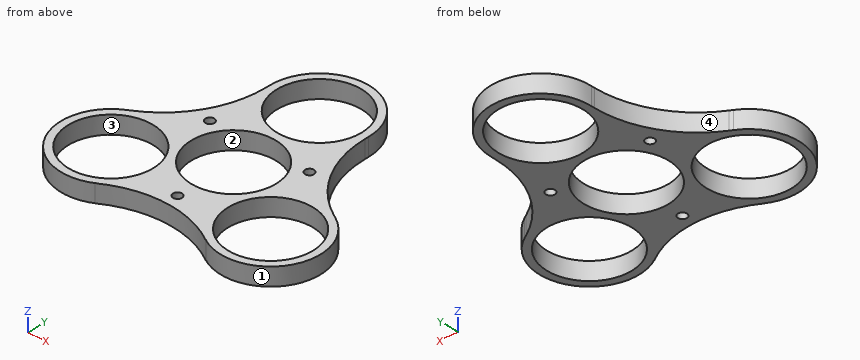
```python
from build123d import *

# Parameters (mm, degrees)
SKETCH1_R           = 11.9
SKETCH1_R_2         = 1.25
BOSS_EXTRUDE1_DEPTH = 2.5


with BuildPart() as part:
    # Sketch1 → Boss-Extrude1 (new, symmetric)
    with BuildSketch(Plane.XY):
        with BuildLine():
            Line((13.998405034, 25.788679153), (13.997620563, 24.84501718))
            ThreePointArc((13.997620563, 24.84501718), (17.915653408, 10.264281088), (28.632025365, -0.370953675))
            Line((28.632025365, -0.370953675), (29.451770584, -0.838410955))
            ThreePointArc((29.451770584, -0.838410955), (34.50421589, -20.231771272), (14.992592767, -24.806286663))
            Line((14.992592767, -24.806286663), (15.585568871, -25.184186379))
            ThreePointArc((15.585568871, -25.184186379), (0, -20.640065896), (-15.585568871, -25.184186379))
            Line((-15.585568871, -25.184186379), (-14.992592767, -24.806286663))
            ThreePointArc((-14.992592767, -24.806286663), (-34.504073282, -20.232007658), (-29.452250217, -0.838684477))
            Line((-29.452250217, -0.838684477), (-28.632523434, -0.371194867))
            ThreePointArc((-28.632523434, -0.371194867), (-17.951478652, 10.204474397), (-13.999324478, 24.706542367))
            Line((-13.999324478, 24.706542367), (-13.995629252, 25.650197431))
            ThreePointArc((-13.995629252, 25.650197431), (-0.069254769, 39.999828705), (13.998405034, 25.788679153))
        make_face()
        Circle(SKETCH1_R, mode=Mode.SUBTRACT)
        with Locations((0, 26)):
            Circle(SKETCH1_R, mode=Mode.SUBTRACT)
        with Locations((22.516660498, -13)):
            Circle(SKETCH1_R, mode=Mode.SUBTRACT)
        with Locations((-22.516660498, -13)):
            Circle(SKETCH1_R, mode=Mode.SUBTRACT)
        with Locations((13.983602476, 7.982266036)):
            Circle(SKETCH1_R_2, mode=Mode.SUBTRACT)
        with Locations((0, -17)):
            Circle(SKETCH1_R_2, mode=Mode.SUBTRACT)
        with Locations((-14.064993078, 7.936657484)):
            Circle(SKETCH1_R_2, mode=Mode.SUBTRACT)
    extrude(amount=BOSS_EXTRUDE1_DEPTH, both=True)


solid = part.part
```
Could you check a few things on this model? Use its own coordinates, in mm. Face numbers are marked on the shaded views. Round coordinates to 2 decimals unless told otherwise and drop trailing zeros. Loops run counter-clockwise (first coordinate to the right, second up) from the corner with the lowest first, then second, coordinate; pieces in that order, holes last. Notation, with made-up numbers: (70, -31.5) - (75, -31.5) arc R24 cw to (75, -12.5) - close; hole circle Ø5 at (12.25, -36). An arc over 180 degrees is marked (long way). Answer in a Markdown table with one row per item. Add a question column.
(1) If we section it at A-A (x = 0): Please give me the cut outline in (y, z), plus the area to 3 significant figures.
(2) I need wall thicknesses on line 1 along Y through (x, z) = (6, -0.85); line 2 along Y through (x, z) = (0, 1.2); line 3 along Y through (x, z) = (-9, -2.2). Which ranges of each line are inside material? Lowest first, please.
(3) If we mould it in two halves opening along Y, with no side actions, what happens to the marked faces 1, 2, 3 and 4? For each: pulls with the +Y half, pulls with the -Y half, needs draft (parallel to the pull), parting line crosses it, or undercut.
(4) If we section it at D-D (x = 22): Please give me the cut outline in (y, z), plus the area to 3 significant figures.
(5) If we section it at B-B (y = -13): Please give me the cut outline in (x, z), plus the area to 3 significant figures.
(6) If we section it at C-C (y = -3): Please give me the cut outline in (x, z).
(7) I'm going to push flat-ended pins straight in: pin 1 (21.5 mm diameter, centred on x = 22.52, y = -13, fed in from +Z); pin 2 (3 mm diameter, centred on y = 23, z = -2, fed in from -X). Where does each tip first touch, or does it pass through?
Model answer:
| question | item | result |
|---|---|---|
| 1 | outline | (-20.64, -2.5) - (-18.25, -2.5) - (-18.25, 2.5) - (-20.64, 2.5) - close; (-15.75, -2.5) - (-11.9, -2.5) - (-11.9, 2.5) - (-15.75, 2.5) - close; (11.9, -2.5) - (14.1, -2.5) - (14.1, 2.5) - (11.9, 2.5) - close; (37.9, -2.5) - (40, -2.5) - (40, 2.5) - (37.9, 2.5) - close |
| 1 | area | 52.7 mm² |
| 2 | line 1 | y = -21.27 to -10.28, 10.28 to 15.72, 36.28 to 38.65 |
| 2 | line 2 | y = -20.64 to -18.25, -15.75 to -11.9, 11.9 to 14.1, 37.9 to 40 |
| 2 | line 3 | y = -22.07 to -7.79, 7.79 to 18.21, 33.79 to 36.72 |
| 3 | face 1 | parting line crosses it |
| 3 | face 2 | undercut |
| 3 | face 3 | undercut |
| 3 | face 4 | pulls with the +Y half |
| 4 | outline | (-26.99, -2.5) - (-24.89, -2.5) - (-24.89, 2.5) - (-26.99, 2.5) - close; (-1.11, -2.5) - (4.82, -2.5) - (4.82, 2.5) - (-1.11, 2.5) - close |
| 4 | area | 40.2 mm² |
| 5 | outline | (-36.52, -2.5) - (-34.42, -2.5) - (-34.42, 2.5) - (-36.52, 2.5) - close; (-10.62, -2.5) - (10.62, -2.5) - (10.62, 2.5) - (-10.62, 2.5) - close; (34.42, -2.5) - (36.52, -2.5) - (36.52, 2.5) - (34.42, 2.5) - close |
| 5 | area | 127 mm² |
| 6 | outline | (-32.31, -2.5) - (-28.97, -2.5) - (-28.97, 2.5) - (-32.31, 2.5) - close; (-16.07, -2.5) - (-11.52, -2.5) - (-11.52, 2.5) - (-16.07, 2.5) - close; (11.52, -2.5) - (16.07, -2.5) - (16.07, 2.5) - (11.52, 2.5) - close; (28.97, -2.5) - (32.31, -2.5) - (32.31, 2.5) - (28.97, 2.5) - close |
| 7 | pin 1 | passes through |
| 7 | pin 2 | stops at x = -14.19 |
